```python
from build123d import *

# Parameters (mm, degrees)
F0_R     = 17.628013
F1_DEPTH = 52.07
F6_DEPTH = 14.986
F2_W     = 34.678817
F2_H     = 55.124529
F7_DEPTH = 9.906
F8_R     = 4.510696
F9_DEPTH = 2514.6


with BuildPart() as f1:
    # F0 (on Front) → F1 (new body)
    with BuildSketch(Plane.XZ):
        Circle(F0_R)
    extrude(amount=F1_DEPTH)

    # F4 (on face) → F6 (join)
    with BuildSketch(Plane.XZ.offset(52.07)):
        with BuildLine():
            ThreePointArc((17.29034, 54.155942), (17.290353, 54.143466), (17.290358, 54.13099))
            ThreePointArc((17.290358, 54.13099), (-0.012476, 36.840637), (-17.29034, 54.155942))
            Line((-17.29034, 54.155942), (-17.628013, 54.155942))
            Line((-17.628013, 54.155942), (-17.628013, 0))
            ThreePointArc((-17.628013, 0), (-1.404154, 17.572), (17.404318, 2.799385))
            Line((17.404318, 2.799385), (17.404318, 54.155942))
            Line((17.404318, 54.155942), (17.29034, 54.155942))
        make_face()
    extrude(amount=-F6_DEPTH)

    # F5 (on face) + F2 (on Front) → F7 (join)
    with BuildSketch(Plane.XZ):
        with BuildLine():
            ThreePointArc((14.317841, 53.7648), (-0.680686, 40.781741), (-14.384703, 55.124529))
            Line((-14.384703, 55.124529), (-20.360976, 55.124529))
            Line((-20.360976, 55.124529), (-20.360976, 0))
            Line((-20.360976, 0), (14.317841, 0))
            Line((14.317841, 0), (14.317841, 53.7648))
        make_face()
    with BuildSketch(Plane.XZ):
        with Locations((-3.021568, 27.562264)):
            Rectangle(F2_W, F2_H)
    extrude(amount=F7_DEPTH)

    # F8 (on face) → F9 (cut)
    with BuildSketch(Plane.XZ.offset(52.07)):
        with Locations((-2.881597, 30.884339)):
            Circle(F8_R)
    extrude(amount=-F9_DEPTH, mode=Mode.SUBTRACT)


solid = f1.part
```
Geometry check sheet. Reference: the model listing, model coordinates, mm. A direction names the side the tool comes from. Coordinates: 2 decimals unless noted, no trailing zeros. Order: outer loops, then holes, each group sorted by start corner. A loop starts at its lowest first (then second) coordinate and runs counter-clockwise, first axis right, second up.
Q1. Draft check along Z on faces 6 (the face through (-3.86, -44.68, 26.48)), 7 (the face through (17.404, -45, 28)), 8 (the face through (8.13, -25.67, -15.64)). Enter one of: released by +Z, released by -Z, zero draft, split by the parting line, or undercut.
Reply:
face 6: undercut
face 7: zero draft
face 8: split by the parting line
Q2. Thickness scan on probe 1 along Y at (x, z) = (-16, 35.5); probe 2 along Y at (x, z) = (6, 38); probe 3 along X at (y, z) = (-42, 5). Record the ranges inside material, lowest first.
Reply:
probe 1: y = -52.07 to -37.08, -9.91 to 0
probe 2: y = -9.91 to 0
probe 3: x = -17.63 to 17.4
Q3. Depth check by flat-ended pin: pin 1 Ø0.7 at (y, z) = (-6.5, 54.5) entering from +X; pin 2 Ø1 at (y, z) = (-30.5, 4) entering from +X; pin 3 Ø16.5 at (y, z) = (-46.5, 29) entering from +X; pin 4 Ø8 at (x, z) = (-2.88, 30.88) entering from +Y. Enter the tip coordinate at first touch or a pass-through.
Reply:
pin 1: stops at x = 14.32
pin 2: stops at x = 17.28
pin 3: stops at x = 17.4
pin 4: passes through
Q4. Sectioned sample at D-D on x = 0. Record the cut outline in (y, z).
Reply:
outline: (-52.07, -17.63) - (0, -17.63) - (0, 27.41) - (-9.91, 27.41) - (-9.91, 17.63) - (-37.08, 17.63) - (-37.08, 27.41) - (-52.07, 27.41) - close; (-52.07, 34.35) - (-37.08, 34.35) - (-37.08, 36.84) - (-52.07, 36.84) - close; (-9.91, 34.35) - (0, 34.35) - (0, 55.12) - (-9.91, 55.12) - close
Q5. Sectioned sample at A-A on z = 24. Record the cut outline in (x, y).
Reply:
outline: (-20.36, -9.91) - (14.32, -9.91) - (14.32, 0) - (-20.36, 0) - close; (-17.63, -52.07) - (17.4, -52.07) - (17.4, -37.08) - (-17.63, -37.08) - close
Q6. Tool access check on faces 1 (the face through (-17.628, -45, 27)), 2 (the face through (0, -52.07, 11)), 3 (the face through (-2, 0, 19)), 4 (the face through (14.318, -5, 32)), 5 (the face through (-19, -5, 0)). Record the directions out of +Z, -Z, +X, -X, +Y, -Y that give a thin tool (end or side, any length) a straight path to the whole face; none if there is none.
Reply:
face 1: +Z, -Z, -X, -Y
face 2: +Z, -Z, +X, -X, -Y
face 3: +Z, -Z, +X, -X, +Y
face 4: +Z, +X, +Y
face 5: -Z, -X, +Y, -Y
Q7. Sectioned sample at B-B on z = 42. Record the cut outline in (x, y), and give its area (3 significant figures).
Reply:
outline: (-20.36, -9.91) - (14.32, -9.91) - (14.32, 0) - (-20.36, 0) - close; (-17.63, -52.07) - (-12.32, -52.07) - (-12.32, -37.08) - (-17.63, -37.08) - close; (12.32, -52.07) - (17.4, -52.07) - (17.4, -37.08) - (12.32, -37.08) - close
area: 499 mm2
